Work out the finished part from the listing and answer in its coordinate system (mm). Face numbers are marked on the shaded views. A direction names the side the tool comes from. Round coordinates to 2 decimals unless told otherwise and drop trailing zeros. Loops run counter-clockwise (first coordinate to the right, second up) from the corner with the lowest first, then second, coordinate; pieces in that order, holes last. Notation, with made-up numbers: (28, -14.75) - (82, -14.75) arc R25 ccw to (82, 11.25) - close; hole circle Ø7 at (79.5, -30). An arc over 180 degrees is marked (long way). Use CSV: the item, a comma, the result in double quotes. Start each with the question number.
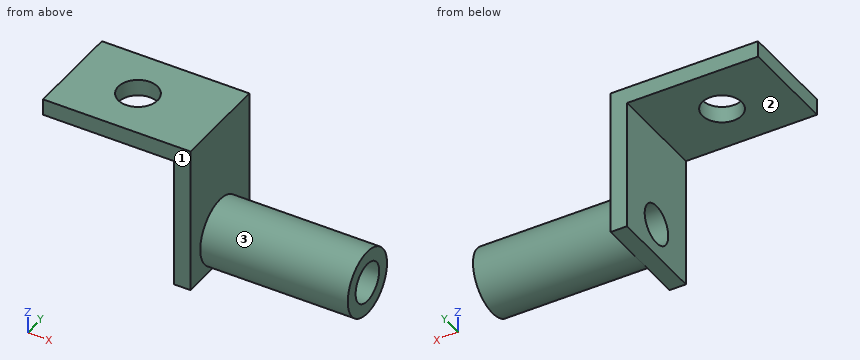
from build123d import *

# Parameters (mm, degrees)
BOSS_EXTRUDE2_DEPTH = 15
SKETCH4_R           = 3
CUT_EXTRUDE2_DEPTH  = 34.634060118
SKETCH7_R           = 5
SKETCH7_R_2         = 3
BOSS_EXTRUDE5_DEPTH = 25
SKETCH8_R           = 3
CUT_EXTRUDE3_DEPTH  = 36.178118199


with BuildPart() as part:
    # Sketch3 → Boss-Extrude2 (new body)
    with BuildSketch(Plane(origin=(0, 0, 0), x_dir=(1, 0, 0), z_dir=(0, 1, 0))):
        Polygon((0, 0), (22.5, 0), (22.5, 22.5), (20, 22.5), (20, 2.5), (0, 2.5), align=None)
    extrude(amount=BOSS_EXTRUDE2_DEPTH)

    # Sketch4 → Cut-Extrude2 (cut, through all)
    with BuildSketch(Plane(origin=(0, 0, -2.5), x_dir=(-1, 0, 0), z_dir=(0, 0, -1))):
        with Locations((-10, 7.5)):
            Circle(SKETCH4_R)
    extrude(amount=-CUT_EXTRUDE2_DEPTH, mode=Mode.SUBTRACT)

    # Sketch7 → Boss-Extrude5 (add)
    with BuildSketch(Plane.ZY.offset(-20)):
        with Locations((-17.5, 7.5)):
            Circle(SKETCH7_R)
        with Locations((-17.5, 7.5)):
            Circle(SKETCH7_R_2, mode=Mode.SUBTRACT)
    extrude(amount=-BOSS_EXTRUDE5_DEPTH)

    # Sketch8 → Cut-Extrude3 (cut, through all)
    with BuildSketch(Plane(origin=(22.5, 0, 0), x_dir=(0, 0, -1), z_dir=(1, 0, 0))):
        with Locations(Location((17.5, 7.5, 0), (0, 0, 180))):
            Circle(SKETCH8_R)
    extrude(amount=-CUT_EXTRUDE3_DEPTH, mode=Mode.SUBTRACT)


solid = part.part
Item 1: Each of these flat-tipped pins is pushed along its axis until it touches: pin 1 Ø10 at (x, z) = (35, -14.5) entering from -Y; pin 2 Ø1.5 at (x, y) = (17, 9.5) entering from -Z; pin 3 Ø4 at (y, z) = (6, -5) entering from -X. Where does it stop, or does it pass through?
Item 2: Find the intervals of material crossed by probe 1 along Y at (x, z) = (10, -0.55); probe 2 along Z at (x, y) = (38, 7.5); probe 3 along Y at (x, z) = (39.75, -17.5), in increasing order. Write a range as [from, to].
Item 3: A cutting plane is placed at D-D (z = -13.5). Determine the outline of the cut face in (x, y).
Item 4: A cutting plane is placed at B-B (z = -17.5). Determine the outline of the cut face in (x, y), plus the area to 4 significant figures.
Item 5: A cutting plane is placed at A-A (x = 10). Determine the outline of the cut face in (y, z).
Item 6: Which of the six approach directions +Z, -Z, +X, -X, +Y, -Y give full straight-line access (tool end or side, diameter ignored) to the marked faces 1, 2 and 3?
Item 7: A cutting plane is placed at C-C (y = 13.25). Determine the outline of the cut face in (x, z).
Result sheet:
1,pin 1,"y = 2.5"
1,pin 2,"z = -2.5"
1,pin 3,"x = 20"
2,probe 1,"[0, 4.5], [10.5, 15]"
2,probe 2,"[-22.5, -20.5], [-14.5, -12.5]"
2,probe 3,"[2.5, 4.5], [10.5, 12.5]"
3,outline,"(20, 0) - (22.5, 0) - (22.5, 4.5) - (45, 4.5) - (45, 10.5) - (22.5, 10.5) - (22.5, 15) - (20, 15) - close"
4,outline,"(20, 0) - (22.5, 0) - (22.5, 2.5) - (45, 2.5) - (45, 4.5) - (20, 4.5) - close; (20, 10.5) - (45, 10.5) - (45, 12.5) - (22.5, 12.5) - (22.5, 15) - (20, 15) - close"
4,area,"112.5 mm^2"
5,outline,"(0, -2.5) - (4.5, -2.5) - (4.5, 0) - (0, 0) - close; (10.5, -2.5) - (15, -2.5) - (15, 0) - (10.5, 0) - close"
6,face 1,"+Z, -Z, +X, -X, -Y"
6,face 2,"-Z, -X, +Y, -Y"
6,face 3,"+X"
7,outline,"(0, -2.5) - (20, -2.5) - (20, -22.5) - (22.5, -22.5) - (22.5, 0) - (0, 0) - close"
